Here's how the part is built. I have some questions about the finished solid (model axes, mm). A direction names the side the tool comes from. Round coordinates to 2 decimals unless told otherwise and drop trailing zeros. Order: outer loops, then holes, each group sorted by start corner. A loop starts at its lowest first (then second) coordinate and runs counter-clockwise, first axis right, second up. Notation, with made-up numbers: (83.5, 83) - (107.5, 83) arc R36 ccw to (107.5, 122) - close; hole circle Ø5 at (-6, 57). An arc over 180 degrees is marked (long way). One line per item, written item: value.
from build123d import *

# Parameters (mm, degrees)
F0_W     = 140
F0_H     = 140
F1_DEPTH = 19
F3_DEPTH = 20
F4_R     = 3


# Not quite as in the source:
# - a feature names something its author has since deleted; it is built from what else it names


with BuildPart() as f1:
    # F0 (on Top) → F1 (new body)
    with BuildSketch(Plane.XY):
        Rectangle(F0_W, F0_H)
    extrude(amount=F1_DEPTH)

    # F2 (on face) → F3 (cut)
    with BuildSketch(Plane.XY.offset(19)):
        Polygon((20, 0), (0, 0), (-5, 0), (-32.2085873907, 37.4088223177), (-55, 21.1437827766), (-10, -45), (50, -38), (50, 45), (20, 45), align=None)
    extrude(amount=-F3_DEPTH, mode=Mode.SUBTRACT)

    # F4
    f4_edges = [f1.edges().sort_by_distance(p)[0] for p in [
        (50, -38, 9.5),
        (50, 45, 9.5),
        (20, 45, 9.5),
        (20, 0, 9.5),
        (-55, 21.143783, 9.5),
        (-10, -45, 9.5),
        (-32.208587, 37.408822, 9.5),
    ]]
    fillet(f4_edges, radius=F4_R)


solid = f1.part
Q1. If we section it at B-B, the plane y = -2.5: Please give me the cut outline in (x, z), then the cut area to 3 significant figures.
Results list:
outline: (-70, 0) - (-38.91, 0) - (-38.91, 19) - (-70, 19) - close; (50, 0) - (70, 0) - (70, 19) - (50, 19) - close
area: 971 mm²
Q2. If we section it at C-C, the plane z = 3: Please give me the cut outline in (x, y).
Results list:
outline: (-70, -70) - (70, -70) - (70, 70) - (-70, 70) - close; hole (-53.35, 18.72) - (-11.02, -43.5) arc R3 ccw to (-8.19, -44.79) - (47.35, -38.31) arc R3 ccw to (50, -35.33) - (50, 42) arc R3 ccw to (47, 45) - (23, 45) arc R3 ccw to (20, 42) - (20, 3) arc R3 cw to (17, 0) - (-5, 0) - (-30.46, 35) arc R3 ccw to (-34.63, 35.68) - (-52.61, 22.85) arc R3 ccw to start
Q3. If we section it at A-A, the plane x = 32: Please give me the cut outline in (y, z).
Results list:
outline: (-70, 0) - (-40.1, 0) - (-40.1, 19) - (-70, 19) - close; (45, 0) - (70, 0) - (70, 19) - (45, 19) - close
Q4. Which directions (+Z, -Z, +X, -X, +Y, -Y) give clear straight access to the entire face, cutting with the end or side of a thin tool? Please do faces 1 (the flat face through (19.188, -41.595, 9.633)), 2 (the flat face through (-1, 1, 0)).
Results list:
face 1: +Z, -Z
face 2: -Z, +X, -X, +Y, -Y
Q5. If I drill on line 1 along X through (y, z) = (4, 15); line 2 along X through (y, z) = (40, 7.5); line 3 along X through (y, z) = (29.5, 7.5), over which ranges is the centre line in solid material (lowest first)?
Results list:
line 1: -70 to -43.34, -7.91 to 20, 50 to 70
line 2: -70 to 20, 50 to 70
line 3: -70 to -43.29, -26.46 to 20, 50 to 70
Q6. We'd pull the mould along Y, two halves only. Please class faces 3 (the cylindrical face through (-32.4, 36.2, 9.4)), 4 (the flat face through (50, 3, 10)), 5 (the flat face through (-70, -1, 9)), 6 (the flat face through (-1, -70, 9)): released by +Y, released by -Y, zero draft, split by the parting line, or undercut.
Results list:
face 3: undercut
face 4: undercut
face 5: zero draft
face 6: released by -Y
